Study the drawing (mm; zero at the part's minimum x, y, z) and answer. Round coordinates to 2 decimals unless told otherwise and drop trailing zeros. Loops run counter-clockwise (first coordinate to the right, second up) from the corner with the lowest first, then second, coordinate; pieces in that order, holes last. Notation, with made-up numbers: (-26, 70.5) -> (8, 70.5) arc R22 ccw to (8, 107.5) -> close; hole circle Ø8 at (21, -7). An arc over 180 degrees is marked (long way). Use one line per item in the form item = value.
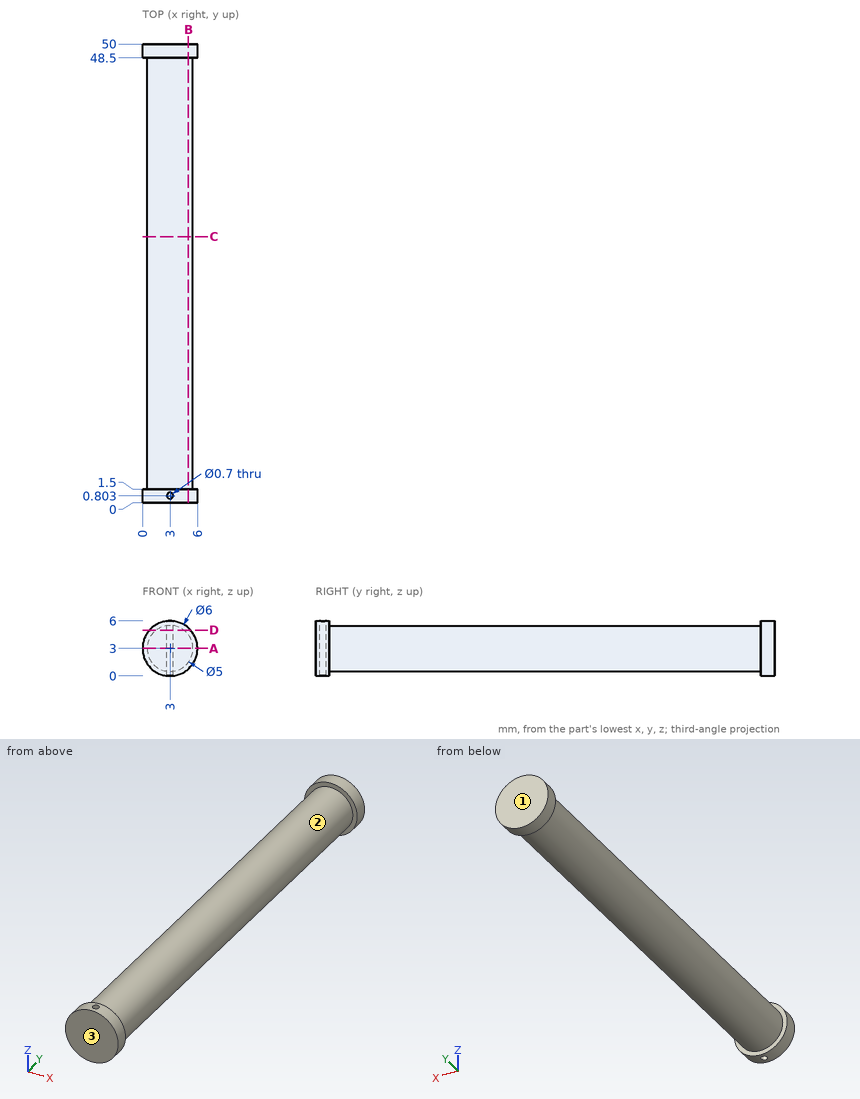
(1) Find section C-C, the plane y = 29. Write down the section's boundary in (x, z).
Completed:
outline = circle Ø5 at (3, 3)
(2) Consider L1, parallel to Y at x = 3, z = 4.75; L2, parallel to Y at x = 2, z = 5.5; L3, parallel to Z at x = 3, y = 11. Determine where each line is inside the solid, lowest interval first.
Completed:
L1 = 0 to 0.45, 1.15 to 50
L2 = 0 to 1.5, 48.5 to 50
L3 = 0.5 to 5.5
(3) Find section A-A, the plane z = 3. Write down the section's boundary in (x, y), then the cut area to 3 significant figures.
Completed:
outline = (0, 0) -> (6, 0) -> (6, 1.5) -> (5.5, 1.5) -> (5.5, 48.5) -> (6, 48.5) -> (6, 50) -> (0, 50) -> (0, 48.5) -> (0.5, 48.5) -> (0.5, 1.5) -> (0, 1.5) -> close; hole circle Ø0.7 at (3, 0.8)
area = 253 mm2
(4) Given P1, Ø1, axis at y = 33.5, z = 1.5, coming from the -X side; P2, Ø2, axis at y = 37, z = 1.5, coming from the +X side; P3, Ø1, axis at x = 0.5, y = 40, coming from the +Z side, each flat-ended and moving along its own axis, determine where each tip first touches the part or whether it passes through.
Completed:
P1 = 0.71
P2 = 5.45
P3 = 4.5
(5) Find section D-D, the plane z = 5. Write down the section's boundary in (x, y).
Completed:
outline = (0.76, 0) -> (5.24, 0) -> (5.24, 1.5) -> (4.5, 1.5) -> (4.5, 48.5) -> (5.24, 48.5) -> (5.24, 50) -> (0.76, 50) -> (0.76, 48.5) -> (1.5, 48.5) -> (1.5, 1.5) -> (0.76, 1.5) -> close; hole circle Ø0.7 at (3, 0.8)
(6) Find section B-B, the plane x = 5. Write down the section's boundary in (y, z).
Completed:
outline = (0, 0.76) -> (1.5, 0.76) -> (1.5, 1.5) -> (48.5, 1.5) -> (48.5, 0.76) -> (50, 0.76) -> (50, 5.24) -> (48.5, 5.24) -> (48.5, 4.5) -> (1.5, 4.5) -> (1.5, 5.24) -> (0, 5.24) -> close
(7) For a pull along Y with two mould halves and no side action, classify the marked faces 1, 2 and 3 as +Y half, -Y half, draft (parallel to the pull), parting line (faces both ways), or undercut.
Completed:
face_1 = +Y half
face_2 = undercut
face_3 = -Y half
